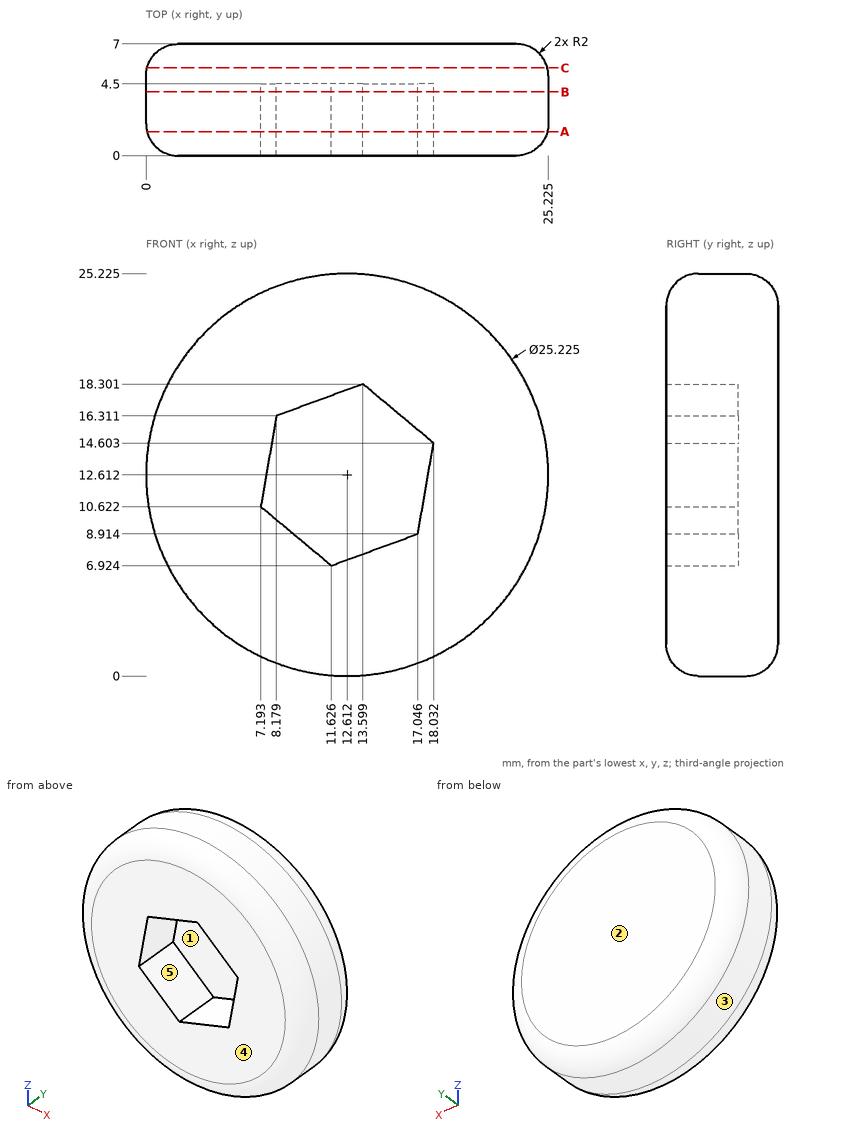
Geometry check sheet. Reference: drawing and pictorial views, mm from the part's lowest x, y, z. A direction names the side the tool comes from. Coordinates: 2 decimals unless noted, no trailing zeros. Order: outer loops, then holes, each group sorted by start corner. A loop starts at its lowest first (then second) coordinate and runs counter-clockwise, first axis right, second up. Notation, with made-up numbers: M 54,-16 L 94,-16 A9 ccw 94,-10 Z; hole C -1.75,25.25 d3. An arc over 180 degrees is marked long. Return JSON: item names as keys, results as strings.
1) Access from +Z, -Z, +X, -X, +Y, -Y to the whole of each face (thin tool, end or side, straight path). Record for the marked faces 4 and 5.
Answer list:
{"face 4": "+Z, -Z, +X, -X, -Y", "face 5": "-Y"}
2) Release check for a two-part mould opening along Z. For the marked faces 1, 2 and 3 record: +Z half, -Z half, draft (parallel to the pull), parting line (faces both ways), or undercut.
Answer list:
{"face 1": "undercut", "face 2": "draft", "face 3": "parting line"}
3) Thickness scan on L1, parallel to X at y = 2, z = 13 (1 decimal); L2, parallel to Z at x = 9, y = 1 (1 decimal); L3, parallel to Z at x = 10.75, y = 3.25 (1 decimal). Record the ranges inside material, lowest first. Write a range as [from, to].
Answer list:
{"L1": "[0, 7.6], [17.8, 25.2]", "L2": "[0.8, 9.1], [16.6, 24.4]", "L3": "[0.1, 7.7], [17.3, 25.1]"}
4) Gauge pin test, flat ends, axial feed: pin 1 (2 mm diameter, centred on y = 4.5, z = 12, fed in from -X); pin 2 (1 mm diameter, centred on x = 5, y = 5.5, fed in from +Z) (1 decimal); pin 3 (3.5 mm diameter, centred on x = 12, z = 10.5, fed in from -Y); pin 4 (2 mm diameter, centred on x = 4.5, y = 4.5, fed in from -Z). Record the tip position at first contact, or that the pin passes through.
Answer list:
{"pin 1": "x = 0", "pin 2": "z = 23", "pin 3": "y = 4.5", "pin 4": "z = 2.2"}
5) Cross-section at C-C, the plane y = 5.5. Record the boundary of the cut face in (x, z).
Answer list:
{"outline": "C 12.61,12.61 d25.1"}
6) Cross-section at B-B, the plane y = 4. Record the boundary of the cut face in (x, z) (1 decimal).
Answer list:
{"outline": "C 12.6,12.6 d25.2; hole M 7.2,10.6 L 11.6,6.9 L 17,8.9 L 18,14.6 L 13.6,18.3 L 8.2,16.3 Z"}
7) Cross-section at A-A, the plane y = 1.5. Record the boundary of the cut face in (x, z) (1 decimal).
Answer list:
{"outline": "C 12.6,12.6 d25.1; hole M 7.2,10.6 L 11.6,6.9 L 17,8.9 L 18,14.6 L 13.6,18.3 L 8.2,16.3 Z"}
